Autodesk Inventor part; units mm, degrees
ref_plane "Work Plane1" through (0, 2.5, 0) normal (0, -1, 0) x (1, 0, 0)
ref_plane "YZ Plane" through (0, 0, 0) normal (1, 0, 0) x (0, 1, 0)
ref_plane "XZ Plane" through (0, 0, 0) normal (0, 1, 0) x (-1, 0, 0)
sketch "Sketch1" plane through (0, 0, 0) normal (0, 1, 0) x (-1, 0, 0)
  line L0 (28, 75) -> (-28, 75)
  line L1 (-28, 75) -> (-28, -75)
  line L2 (-28, -75) -> (28, -75)
  line L3 (28, -75) -> (28, 75)
  line L4 (28, 75) -> (-28, -75) construction
  line L5 (-28, 75) -> (28, -75) construction
  point P0 (0, 0)
  dimension "d0" = 56
  dimension "d1" = 150
extrude "Extrusion1" add sketch "Sketch1" along normal blind 5
sketch "Sketch2" plane through (0, 5, 0) normal (0, 1, 0) x (1, 0, 0)
  line L0 (-28, 12.5) -> (-25, 12.5)
  line L1 (-25, 12.5) -> (-25, -12.5)
  line L2 (-25, -12.5) -> (-28, -12.5)
  line L3 (-28, -12.5) -> (-28, 12.5)
  line L4 (-28, 75) -> (-28, -75)
  line L5 (0, 0) -> (0, 30.0888)
  line L6 (28, 12.5) -> (25, 12.5)
  line L7 (25, 12.5) -> (25, -12.5)
  line L8 (25, -12.5) -> (28, -12.5)
  line L9 (28, -12.5) -> (28, 12.5)
  point P0 (-28, 0)
  dimension "d4" = 3
  dimension "d5" = 25
extrude "Extrusion2" add sketch "Sketch2" along normal blind 80
sketch "Sketch3" plane through (28, 0, 75) normal (1, 0, 0) x (0, 0, -1)
  circle A0 centre (66.65, 55) radius 1.75
  circle A1 centre (66.65, 80) radius 1.75
  circle A2 centre (83.35, 80) radius 1.75
  circle A3 centre (83.35, 55) radius 1.75
  circle A4 centre (66.65, 55) radius 1.75
  circle A5 centre (66.65, 80) radius 1.75
  circle A6 centre (83.35, 80) radius 1.75
  circle A7 centre (83.35, 55) radius 1.75
  line L0 (83.35, 55) -> (66.65, 80)
  line L1 (66.65, 80) -> (66.65, 55)
  line L2 (66.65, 55) -> (83.35, 80)
  line L3 (83.35, 80) -> (83.35, 55)
  line L4 (66.65, 55) -> (83.35, 55)
  line L5 (83.35, 80) -> (66.65, 80)
  line L6 (0, 0) -> (150, 0)
  line L7 (150, 0) -> (150, 5)
  line L8 (87.5, 5) -> (150, 5)
  line L9 (87.5, 5) -> (87.5, 85)
  line L10 (62.5, 85) -> (87.5, 85)
  line L11 (62.5, 5) -> (62.5, 85)
  line L12 (0, 5) -> (62.5, 5)
  line L13 (0, 0) -> (0, 5)
  line L14 (62.5, 80) -> (87.5, 80)
  line L15 (87.5, 5) -> (87.5, 85)
  point P0 (75, 0)
  point P1 (75, 80)
  dimension "d12" = 5
  dimension "d14" = 16.7
  dimension "d15" = 25
extrude "Extrusion3" cut sketch "Sketch3" against normal through all contours L4 L2 A0 | A0 L1 L4 | L2 L1 A0 | L4 L3 A3 | A3 L0 L4 | L1 L0 A1 | A1 L14 L1 | A3 L3 L0 | L0 L5 A1 | L2 L3 A2 | A2 L5 L2 | A1 L5 L14 | A2 L14 L5 | L3 L14 A2
sketch "Sketch4" plane through (-28, 0, 75) normal (0, 0, 1) x (1, 0, 0)
  circle A0 centre (14, 10) radius 2.5
  circle A1 centre (42, 10) radius 2.5
  line L0 (6.5, 5) -> (9, 5)
  line L1 (47, 5) -> (49.5, 5)
  line L2 (47, 10) -> (47, 5)
  arc A2 (47, 10) -> (37, 10) centre (42, 10) ccw
  line L3 (37, 5) -> (37, 10)
  line L4 (19, 5) -> (37, 5)
  line L5 (19, 10) -> (19, 5)
  arc A3 (19, 10) -> (9, 10) centre (14, 10) ccw
  line L6 (9, 5) -> (9, 10)
  line L7 (0, 5) -> (56, 5)
  point P0 (28, 0)
  point P1 (33.2021, 4.5034)
  point P2 (28, 5)
  point P3 (9, 5)
  dimension "d18" = 43
  dimension "d19" = 18
  dimension "d20" = 5
  dimension "d21" = 5
  dimension "d22" = 5
  dimension "d23" = 5
  dimension "d24" = 5
  dimension "d25" = 5
extrude "Extrusion4" add sketch "Sketch4" against normal blind 3
ref_plane "Work Plane1" through (0, 2.5, 0) normal (0, -1, 0) x (1, 0, 0)
mirror "Mirror1" about plane through (0, 2.5, 0) normal (0, -1, 0) of "Extrusion4"
mirror "Mirror2" about plane through (0, 0, 0) normal (0, 0, 1) of "Extrusion4", "Mirror1"
sketch "Sketch5" plane through (28, 0, 75) normal (0, 0, 1) x (1, 0, 0)
  line L0 (-47, 5) -> (-56, 5)
  line L1 (0, 5) -> (-9, 5)
  line L2 (-47, 5) -> (-9, 5)
  circle A0 centre (-14, -5) radius 2.5
  circle A1 centre (-42, -5) radius 2.5
  circle A2 centre (-14, 10) radius 2.5
  circle A3 centre (-42, 10) radius 2.5
  line L3 (-56, 0) -> (-47, 0)
  line L4 (-47, -5) -> (-47, 0)
  arc A4 (-47, -5) -> (-37, -5) centre (-42, -5) ccw
  line L5 (-37, 0) -> (-37, -5)
  line L6 (-37, 0) -> (-19, 0)
  line L7 (-19, -5) -> (-19, 0)
  arc A5 (-19, -5) -> (-9, -5) centre (-14, -5) ccw
  line L8 (-9, 0) -> (-9, -5)
  line L9 (-9, 0) -> (0, 0)
  line L10 (0, 0) -> (0, 5)
  line L11 (-9, 5) -> (0, 5)
  line L12 (-9, 5) -> (-9, 10)
  arc A6 (-9, 10) -> (-19, 10) centre (-14, 10) ccw
  line L13 (-19, 10) -> (-19, 5)
  line L14 (-37, 5) -> (-19, 5)
  line L15 (-37, 5) -> (-37, 10)
  arc A7 (-37, 10) -> (-47, 10) centre (-42, 10) ccw
  line L16 (-47, 10) -> (-47, 5)
  line L17 (-56, 5) -> (-47, 5)
  line L18 (-56, 0) -> (-56, 5)
  point P0 (-28, 0)
extrude "Extrusion5" cut sketch "Sketch5" against normal through all contours L16 A7 L15 L2 | L13 A6 L12 L2
properties part number "Mounting atas"
Model file for the job. Use its own axes, mm. A direction names the side the tool comes from. Round coordinates to 2 decimals unless told otherwise and drop trailing zeros. Loops run counter-clockwise (first coordinate to the right, second up) from the corner with the lowest first, then second, coordinate; pieces in that order, holes last. Notation, with made-up numbers: M -22.5,34 L -11.5,34 A28 cw -11.5,57 Z; hole C 4.5,-19.75 d7. An arc over 180 degrees is marked long. One line per question, with ' | ' between items.
1) Band-saw the part on A-A (z = 8.35). Give the cut face in (x, y).
Solved:
outline: M -28,0 L 28,0 L 28,53.25 L 25,53.25 L 25,5 L -25,5 L -25,53.25 L -28,53.25 Z; M -28,56.75 L -25,56.75 L -25,78.25 L -28,78.25 Z; M -28,81.75 L -25,81.75 L -25,85 L -28,85 Z; M 25,56.75 L 28,56.75 L 28,78.25 L 25,78.25 Z; M 25,81.75 L 28,81.75 L 28,85 L 25,85 Z
2) Drill centre lines: line 1 along Z through (x, y) = (26, 80); line 2 along X through (y, z) = (-5, 73.4); line 3 along Y through (x, z) = (-26, 8). Where is each one in solid material? Low to high.
Solved:
line 1: z = -12.5 to -10.1, -6.6 to 6.6, 10.1 to 12.5 | line 2: x = -19 to -16.5, -11.5 to -9, 9 to 11.5, 16.5 to 19 | line 3: y = 0 to 53.29, 56.71 to 78.29, 81.71 to 85
3) Flat gauge pins, fed straight in: pin 1 (4 mm diameter, centred on x = -1, z = -5, fed in from -Y); pin 2 (1.5 mm diameter, centred on x = 26.5, y = 56, fed in from +Z); pin 3 (2.5 mm diameter, centred on y = -1.5, z = 74, fed in from -X). Where does each tip first touch, or does it go through?
Solved:
pin 1: stops at y = 0 | pin 2: stops at z = 12.5 | pin 3: stops at x = -19
4) Band-saw the part on C-C (x = 13). Give the cut face in (y, z).
Solved:
outline: M -9.9,-75 L -7.29,-75 L -7.29,-72 L -9.9,-72 Z; M -9.9,72 L -7.29,72 L -7.29,75 L -9.9,75 Z; M -2.71,-75 L 5,-75 L 5,75 L -2.71,75 L -2.71,72 L 0,72 L 0,-72 L -2.71,-72 Z
5) Band-saw the part on B-B (y = 59). Give the cut face in (x, z), then the cut area to 3 significant figures.
Solved:
outline: M -28,-12.5 L -25,-12.5 L -25,12.5 L -28,12.5 Z; M 25,-12.5 L 28,-12.5 L 28,12.5 L 25,12.5 Z | area: 150 mm²
6) Mould opens along Y. For faces 6 (the flat face through (-14, -2, 72)), 7 (the flat face through (26, 85, 0)), 8 (the cylindrical face through (11.5, -4.9, 73.5)) say: +Y half, -Y half, draft (parallel to the pull), parting line (faces both ways), or undercut.
Solved:
face 6: draft | face 7: +Y half | face 8: undercut
7) Band-saw the part on D-D (z = 47.5). Give the cut face in (x, y).
Solved:
outline: M -28,0 L 28,0 L 28,5 L -28,5 Z
8) 3-axis set-ups, long thin cutter, end or side, ignore diameter. For faces 1 (the flat face through (-26, 44, 12.5)), 2 (the flat face through (-9, -3, -74)), 3 (the flat face through (19, -2, 74)), 4 (the flat face through (-25, 44, 0)), 5 (the flat face through (-19, -3, 74)): which of +Z, -Z, +X, -X, +Y, -Y reach the whole face in a straight line?
Solved:
face 1: +Z, +X, -X, +Y | face 2: +Z, -Z, -Y | face 3: +Z, -Z, +X, -Y | face 4: +Z, -Z, +Y | face 5: +Z, -Z, -X, -Y
